```python
from build123d import *

# Parameters (mm, degrees)
SKETCH_1_R               = 13.75
EXTRUDE_1_DEPTH          = 38
SKETCH_2_R               = 5
EXTRUDE_2_DEPTH          = 2
SKETCH_3_R               = 1.15
EXTRUDE_3_DEPTH          = 13
HOLE_WIZARD_M2_5_1_D     = 2.05
HOLE_WIZARD_M2_5_1_DEPTH = 3.75
HOLE_WIZARD_M2_5_1_TIP   = 0.615882135


with BuildPart() as part:
    # 草图1 → 凸台-拉伸1 (new body)
    with BuildSketch(Plane(origin=(0, 0, 0), x_dir=(1, 0, 0), z_dir=(0, 1, 0))):
        Circle(SKETCH_1_R)
    extrude(amount=EXTRUDE_1_DEPTH)

    # 草图2 → 凸台-拉伸2 (add)
    with BuildSketch(Plane(origin=(0, 38, 0), x_dir=(1, 0, 0), z_dir=(0, 1, 0))):
        Circle(SKETCH_2_R)
    extrude(amount=EXTRUDE_2_DEPTH)

    # 草图3 → 凸台-拉伸3 (add)
    with BuildSketch(Plane(origin=(0, 40, 0), x_dir=(1, 0, 0), z_dir=(0, 1, 0))):
        Circle(SKETCH_3_R)
    extrude(amount=EXTRUDE_3_DEPTH)

    # M2.5 螺纹孔1
    with Locations(Plane(origin=(0, 38, 0), x_dir=(1, 0, 0), z_dir=(0, 1, 0))):
        with Locations((0, 8), (0, -8)):
            Hole(HOLE_WIZARD_M2_5_1_D / 2, depth=HOLE_WIZARD_M2_5_1_DEPTH)
            with Locations((0, 0, -(HOLE_WIZARD_M2_5_1_DEPTH + HOLE_WIZARD_M2_5_1_TIP / 2))):  # 118° drill point
                Cone(0, HOLE_WIZARD_M2_5_1_D / 2, HOLE_WIZARD_M2_5_1_TIP, mode=Mode.SUBTRACT)


solid = part.part
```
Design review of the part built by this model. Coordinates are the model's own, in mm. A direction names the side the tool comes from. Give positions to 0.01 mm unless a question says otherwise; leave off trailing zeros. Loops run counter-clockwise (first coordinate to the right, second up) from the corner with the lowest first, then second, coordinate; pieces in that order, holes last. Notation, with made-up numbers: M 17.25,8 L 27.25,8 A18 ccw 27.25,29 Z; hole C 40.5,-40 d5. An arc over 180 degrees is marked long. Return JSON: item names as keys, results as strings. Group by question number.
Item 1: For probe 1 along Z at (x, y) = (0, 35.85) (3 decimals); probe 2 along Z at (x, y) = (-0.5, 36); probe 3 along X at (y, z) = (36.85, 8) (3 decimals), list the stretches that pass through material, from the lowest coordinate up.
Item 2: We need section D-D (y = 43). Give the boundary of the cut face in (x, z).
Item 3: Tool access review of faces 1 (the cylindrical face through (-2.981, 18.734, 13.423)), 2 (the flat face through (6, 38, 0)): name each direction out of +Z, -Z, +X, -X, +Y, -Y from which nothing blocks a thin tool from reaching the whole face with its end or side.
Item 4: Insertion check: pin 1 Ø2.5 at (x, z) = (0, -8) entering from +Y; pin 2 Ø8 at (x, z) = (5, -3) entering from +Y; pin 3 Ø3 at (x, y) = (-7, 10.5) entering from +Z; pin 4 Ø8 at (x, y) = (-1.5, 7) entering from -Z. Each pin has a flat end and moves straight along its axis. Give the tip position at first contact, or say it passes through.
Item 5: We need section A-A (z = 0). Give the boundary of the cut face in (x, y).
Item 6: Mouldability with a two-part tool opening along Z and no side actions: class faces 3 (the flat face through (0, 53, 0)), 4 (the cylindrical face through (0.76, 36.1, -8.69)), 5 (the cylindrical face through (-0.91, 46.41, 0.7)) as released by +Z, released by -Z, zero draft, split by the parting line, or undercut.
Item 7: We need section B-B (x = 2.75). Give the boundary of the cut face in (y, z).
Item 8: We need section C-C (y = 37). Give the boundary of the cut face in (x, z) (3 decimals).
Output:
{
 "1": {"probe 1": "z = -13.75 to -9.025, -6.975 to 6.975, 9.025 to 13.75", "probe 2": "z = -13.74 to -8.89, -7.11 to 7.11, 8.89 to 13.74", "probe 3": "x = -11.183 to -1.025, 1.025 to 11.183"},
 "2": {"outline": "C 0,0 d2.3"},
 "3": {"face 1": "+Y, -Y", "face 2": "+Y"},
 "4": {"pin 1": "stops at y = 38", "pin 2": "stops at y = 40", "pin 3": "stops at z = 12.6", "pin 4": "stops at z = -13.75"},
 "5": {"outline": "M -13.75,0 L 13.75,0 L 13.75,38 L 5,38 L 5,40 L 1.15,40 L 1.15,53 L -1.15,53 L -1.15,40 L -5,40 L -5,38 L -13.75,38 Z"},
 "6": {"face 3": "zero draft", "face 4": "undercut", "face 5": "split by the parting line"},
 "7": {"outline": "M 0,-13.47 L 38,-13.47 L 38,-4.18 L 40,-4.18 L 40,4.18 L 38,4.18 L 38,13.47 L 0,13.47 Z"},
 "8": {"outline": "C 0,0 d27.5; hole C 0,-8 d2.05; hole C 0,8 d2.05"}
}
